Print and shaded views of the part. All mm, measured from the part's lowest x, y and z. A direction names the side the tool comes from. Coordinates: 2 decimals unless noted, no trailing zeros. Order: outer loops, then holes, each group sorted by start corner. A loop starts at its lowest first (then second) coordinate and runs counter-clockwise, first axis right, second up.
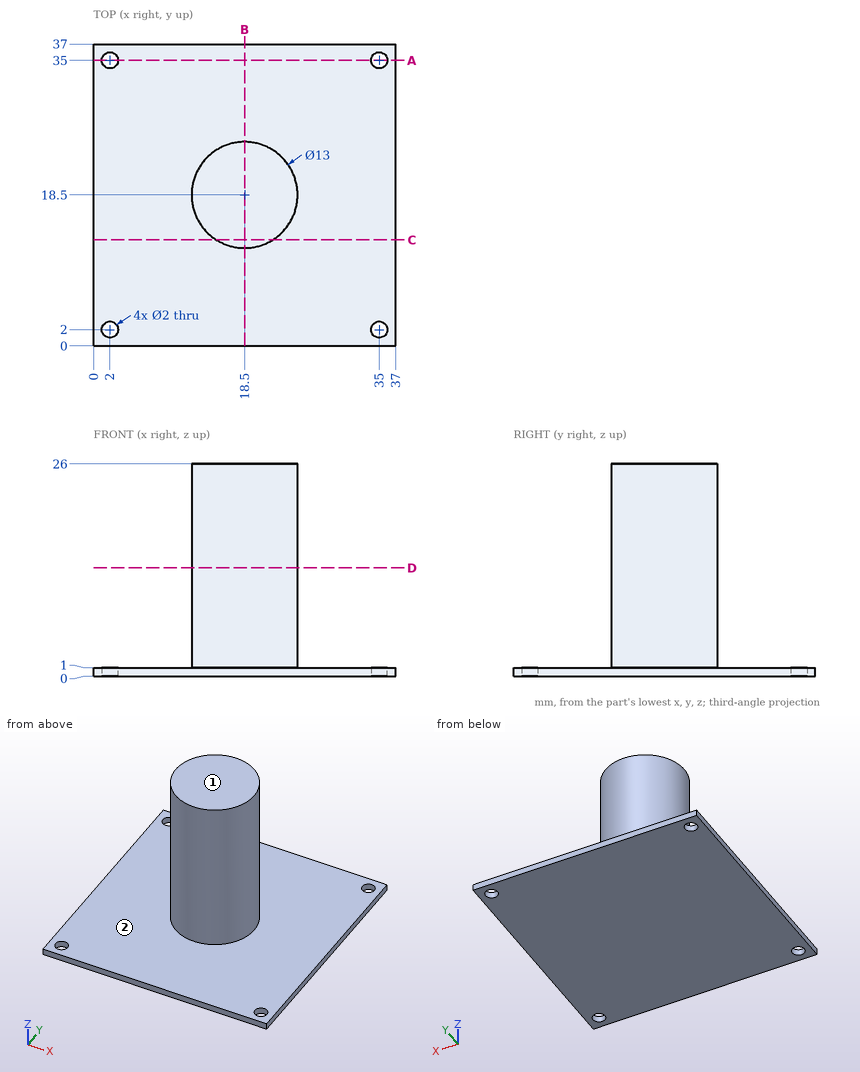
Q1. Probe line 1 (Y direction, x = 35, z = 0.7); line 2 (Z direction, x = 16, y = 33). List the from-to ranges inside material, lowest first.
Established:
line 1: y = 0 to 1, 3 to 34, 36 to 37
line 2: z = 0 to 1
Q2. Cut at B-B, the plane x = 18.5. List the corners of the cut face in (y, z), plus the area to 3 significant figures.
Established:
outline: (0, 0) - (37, 0) - (37, 1) - (25, 1) - (25, 26) - (12, 26) - (12, 1) - (0, 1) - close
area: 362 mm2
Q3. Cut at D-D, the plane z = 13.25. List the corners of the cut face in (x, y).
Established:
outline: circle Ø13 at (18.5, 18.5)
Q4. Which spindle directions (+Z, -Z, +X, -X, +Y, -Y) get a long thin tool onto all of the face, cutting with end or side? Do the marked faces 1 and 2. Say none if no direction does.
Established:
face 1: +Z, +X, -X, +Y, -Y
face 2: +Z
Q5. Cut at A-A, the plane y = 35. List the corners of the cut face in (x, z).
Established:
outline: (0, 0) - (1, 0) - (1, 1) - (0, 1) - close; (3, 0) - (34, 0) - (34, 1) - (3, 1) - close; (36, 0) - (37, 0) - (37, 1) - (36, 1) - close
Q6. Drop flat-ended pins along their axis: P1, Ø3, axis at x = 2, y = 2, coming from the -Z side; P2, Ø10, axis at y = 5.5, z = 13.5, coming from the -X side; P3, Ø1, axis at x = 30, y = 29.5, coming from the +Z side. Give the stop position or say it passes through.
Established:
P1: stops at z = 0
P2: passes through
P3: stops at z = 1
Q7. Cut at C-C, the plane y = 13. List the corners of the cut face in (x, z).
Established:
outline: (0, 0) - (37, 0) - (37, 1) - (21.96, 1) - (21.96, 26) - (15.04, 26) - (15.04, 1) - (0, 1) - close
